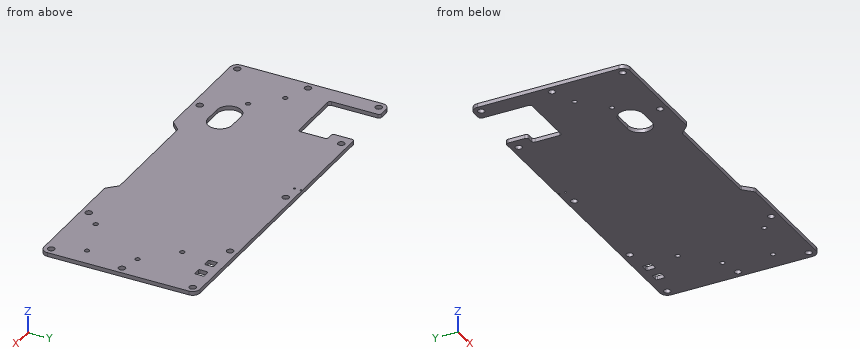
Autodesk Inventor part; units mm, degrees
ref_plane "YZ Plane" through (0, 0, 0) normal (1, 0, 0) x (0, 1, 0)
ref_plane "XZ Plane" through (0, 0, 0) normal (0, 1, 0) x (-1, 0, 0)
ref_plane "XY Plane" through (0, 0, 0) normal (0, 0, 1) x (1, 0, 0)
sketch "Sketch1" plane through (0, 0, 0) normal (0, 0, 1) x (1, 0, 0)
  line L0 (150, 61) -> (150, 3)
  arc A0 (147, 0) -> (150, 3) centre (147, 3) ccw
  line L1 (147, 0) -> (100.4142, 0)
  arc A1 (99.7071, 0.2929) -> (100.4142, 0) centre (100.4142, 1) ccw
  line L2 (99.7071, 0.2929) -> (96.2929, 3.7071)
  arc A2 (96.2929, 3.7071) -> (95.5858, 4) centre (95.5858, 3) ccw
  line L3 (95.5858, 4) -> (51.4142, 4)
  arc A3 (51.4142, 4) -> (50.7071, 3.7071) centre (51.4142, 3) ccw
  line L4 (50.7071, 3.7071) -> (47.2929, 0.2929)
  arc A4 (46.5858, 0) -> (47.2929, 0.2929) centre (46.5858, 1) ccw
  line L5 (46.5858, 0) -> (3, 0)
  arc A5 (0, 3) -> (3, 0) centre (3, 3) ccw
  line L6 (0, 3) -> (0, 61)
  arc A6 (3, 64) -> (0, 61) centre (3, 61) ccw
  line L7 (3, 64) -> (6.5, 64)
  arc A7 (7.5, 63) -> (6.5, 64) centre (6.5, 63) ccw
  line L8 (7.5, 63) -> (7.5, 44)
  arc A8 (7.5, 44) -> (8.5, 43) centre (8.5, 44) ccw
  line L9 (8.5, 43) -> (30.5, 43)
  arc A9 (30.5, 43) -> (31.5, 44) centre (30.5, 44) ccw
  line L10 (31.5, 44) -> (31.5, 54)
  arc A10 (31.5, 54) -> (30.5, 55) centre (30.5, 54) ccw
  line L11 (30.5, 55) -> (28.5, 55)
  arc A11 (27.5, 56) -> (28.5, 55) centre (28.5, 56) ccw
  line L12 (27.5, 56) -> (27.5, 63)
  arc A12 (28.5, 64) -> (27.5, 63) centre (28.5, 63) ccw
  line L13 (28.5, 64) -> (147, 64)
  arc A13 (150, 61) -> (147, 64) centre (147, 61) ccw
  arc A14 (44, 15) -> (39, 20) centre (39, 15) ccw
  arc A15 (39, 10) -> (44, 15) centre (39, 15) ccw
  line L14 (39, 10) -> (32, 10)
  arc A16 (27, 15) -> (32, 10) centre (32, 15) ccw
  arc A17 (32, 20) -> (27, 15) centre (32, 15) ccw
  line L15 (32, 20) -> (39, 20)
  arc A18 (127.8, 60.9) -> (127.3, 60.4) centre (127.8, 60.4) ccw
  line L16 (127.3, 60.4) -> (127.3, 57.6)
  arc A19 (127.3, 57.6) -> (127.8, 57.1) centre (127.8, 57.6) ccw
  line L17 (127.8, 57.1) -> (130.2, 57.1)
  arc A20 (130.2, 57.1) -> (130.7, 57.6) centre (130.2, 57.6) ccw
  line L18 (127.8, 60.9) -> (130.2, 60.9)
  arc A21 (130.7, 60.4) -> (130.2, 60.9) centre (130.2, 60.4) ccw
  line L19 (130.7, 60.4) -> (130.7, 57.6)
  arc A22 (135.3, 60.9) -> (134.8, 60.4) centre (135.3, 60.4) ccw
  line L20 (134.8, 60.4) -> (134.8, 57.6)
  arc A23 (134.8, 57.6) -> (135.3, 57.1) centre (135.3, 57.6) ccw
  line L21 (135.3, 57.1) -> (137.7, 57.1)
  arc A24 (137.7, 57.1) -> (138.2, 57.6) centre (137.7, 57.6) ccw
  line L22 (135.3, 60.9) -> (137.7, 60.9)
  arc A25 (138.2, 60.4) -> (137.7, 60.9) centre (137.7, 60.4) ccw
  line L23 (138.2, 60.4) -> (138.2, 57.6)
  circle A26 centre (68, 60.85) radius 0.4
  circle A27 centre (68, 63.55) radius 0.4
  circle A28 centre (13, 28) radius 1
  circle A29 centre (23, 18) radius 1
  circle A30 centre (126.75, 46) radius 1
  circle A31 centre (138.75, 34) radius 1
  circle A32 centre (3, 61) radius 1.375
  circle A33 centre (32, 61) radius 1.375
  circle A34 centre (118, 61) radius 1.375
  circle A35 centre (147, 61) radius 1.375
  circle A36 centre (147, 3) radius 1.375
  circle A37 centre (118, 3) radius 1.375
  circle A38 centre (32, 3) radius 1.375
  circle A39 centre (3, 3) radius 1.375
  circle A40 centre (3, 32) radius 1.375
  circle A41 centre (75, 61) radius 1.375
  circle A42 centre (124, 9) radius 1
  circle A43 centre (142, 15) radius 1
  circle A44 centre (147, 32) radius 1.375
  point P0 (0, 0)
extrude "Extrusion1" add sketch "Sketch1" along normal blind 1.6
properties part number "pcb"
Could you check a few things on this model? Use its own coordinates, in mm. Round coordinates to 2 decimals unless told otherwise and drop trailing zeros. Loops run counter-clockwise (first coordinate to the right, second up) from the corner with the lowest first, then second, coordinate; pieces in that order, holes last. Notation, with made-up numbers: (4.25, -6) - (61.25, -6) arc R35 ccw to (61.25, 31) - close; hole circle Ø3 at (83.5, 1.25). An arc over 180 degrees is marked (long way). Answer in a Markdown table with one row per item. Add a question column.
(1) If we section it at D-D (z = 1): State how many separate pieces and enclosed holes the cut face has, plus the area to 3 significant figures.
(2) If we section it at C-C (x = 54.5): Please give me the cut outline in (y, z), plus the area to 3 significant figures.
(3) If we section it at A-A (y = 12): Please give me the cut outline in (x, z), plus the area to 3 significant figures.
(4) I need wall thicknesses on line 1 along X through (y, z) = (58, 1.05); line 2 along Y through (x, z) = (118, 1) (3 decimals); line 3 along X through (y, z) = (57, 1.3). Which ranges of each line are inside material? Lowest first, please.
(5) If we section it at B-B (y = 50): Please give me the cut outline in (x, z), plus the area to 3 significant figures.
(6) I'm going to push a flat-ended pin straight in: pin 1 (2 mm diameter, centred on x = 3, y = 3, fed in from +Z). Where does the tip first touch, or does it pass through?
Model answer:
| question | item | result |
|---|---|---|
| 1 | separate pieces | 1 |
| 1 | enclosed holes | 22 |
| 1 | area | 8,670 mm² |
| 2 | outline | (4, 0) - (64, 0) - (64, 1.6) - (4, 1.6) - close |
| 2 | area | 96.0 mm² |
| 3 | outline | (0, 0) - (28, 0) - (28, 1.6) - (0, 1.6) - close; (43, 0) - (150, 0) - (150, 1.6) - (43, 1.6) - close |
| 3 | area | 216 mm² |
| 4 | line 1 | x = 0 to 7.5, 27.5 to 127.3, 130.7 to 134.8, 138.2 to 150 |
| 4 | line 2 | y = 0 to 1.625, 4.375 to 59.625, 62.375 to 64 |
| 4 | line 3 | x = 0 to 7.5, 27.5 to 150 |
| 5 | outline | (0, 0) - (7.5, 0) - (7.5, 1.6) - (0, 1.6) - close; (31.5, 0) - (150, 0) - (150, 1.6) - (31.5, 1.6) - close |
| 5 | area | 202 mm² |
| 6 | pin 1 | passes through |
